Here's how the part is built. I have some questions about the finished solid (model axes, mm). A direction names the side the tool comes from. Give positions to 0.01 mm unless a question says otherwise; leave off trailing zeros. Loops run counter-clockwise (first coordinate to the right, second up) from the corner with the lowest first, then second, coordinate; pieces in that order, holes last.
Q1. For faces 5 (the face through (12, 0, 0)), 6 (the face through (-13.99, 5.99, 2.15)), 7 (the face through (10.907, -10.98, 5.898)), which set-ups out of +Z, -Z, +X, -X, +Y, -Y let a thin tool reach every point of the face, with its end or its side?
Q2. Thinking about a two-plate mould opening in Y: for faces 1 (the face through (0, 0, 7.5)), 2 (the face through (7, -13, 4.25)), 3 (the face through (-1, 13, 4.25)), 4 (the face through (-2.343, 17.847, 3.698)), which applies, pulls with the +Y half, pulls with the -Y half, needs draft (parallel to the pull), parting line crosses it, or undercut?
Q3. Suppose I cut it at D-D (z = -0.5). List the corners of the cut face in (x, y) for me.
Q4. I'm going to push flat-ended pins straight in: P1, Ø2.5, axis at x = 14.5, y = 4.5, coming from the +Z side; P2, Ø3, axis at y = -6, z = 6, coming from the +X side; P3, Ø1, axis at x = -12.5, y = -1.5, coming from the -Z side. Where does each tip first touch, or does it pass through?
Q5. Suppose I cut it at C-C (y = 14.5). List the corners of the cut face in (x, z) for me, and give its area (3 significant figures).
Q6. Suppose I cut it at B-B (y = 0). List the corners of the cut face in (x, z) for me.
Q7. I need wall thicknesses on probe 1 along Y at (x, z) = (0, 1.8); probe 2 along Y at (x, z) = (0, -4); probe 3 along Z at (x, y) = (14.5, -0.5). Which ranges of each line are inside material? Lowest first, please.
Q8. Suppose I cut it at A-A (x = 0). List the corners of the cut face in (y, z) for me.
```python
from build123d import *

# Parameters (mm, degrees)
SKETCH1_R           = 18
BOSS_EXTRUDE1_DEPTH = 7.5
SKETCH2_R           = 11.5
SKETCH2_R_2         = 4.5
BOSS_EXTRUDE2_DEPTH = 7.25
SKETCH3_R           = 1.524
CUT_EXTRUDE1_DEPTH  = 16.75
SKETCH4_R           = 2.5
CUT_EXTRUDE2_DEPTH  = 3.25


with BuildPart() as part:
    # Sketch1 → Boss-Extrude1 (new body)
    with BuildSketch(Plane.XY):
        Circle(SKETCH1_R)
    extrude(amount=BOSS_EXTRUDE1_DEPTH)

    # Sketch2 → Boss-Extrude2 (add)
    with BuildSketch(Plane(origin=(0, 0, 0), x_dir=(-1, 0, 0), z_dir=(0, 0, -1))):
        Circle(SKETCH2_R)
        Circle(SKETCH2_R_2, mode=Mode.SUBTRACT)
    extrude(amount=BOSS_EXTRUDE2_DEPTH)

    # Sketch3 → Cut-Extrude1 (cut)
    with BuildSketch(Plane.XY.offset(7.5)):
        with Locations((0, 14.5)):
            Circle(SKETCH3_R)
        with Locations((13.790319486, 4.480746418)):
            Circle(SKETCH3_R)
        with Locations((8.522886158, -11.730746418)):
            Circle(SKETCH3_R)
        with Locations((-8.522886158, -11.730746418)):
            Circle(SKETCH3_R)
        with Locations((-13.790319486, 4.480746418)):
            Circle(SKETCH3_R)
    extrude(amount=-CUT_EXTRUDE1_DEPTH, mode=Mode.SUBTRACT)

    # Sketch4 → Cut-Extrude2 (cut)
    with BuildSketch(Plane.XY.offset(7.5)):
        with Locations((0, 14.5)):
            Circle(SKETCH4_R)
        with Locations((13.790319486, 4.480746418)):
            Circle(SKETCH4_R)
        with Locations((8.522886158, -11.730746418)):
            Circle(SKETCH4_R)
        with Locations((-8.522886158, -11.730746418)):
            Circle(SKETCH4_R)
        with Locations((-13.790319486, 4.480746418)):
            Circle(SKETCH4_R)
    extrude(amount=-CUT_EXTRUDE2_DEPTH, mode=Mode.SUBTRACT)


solid = part.part
```
Solutions:
1. face 5: -Z
1. face 6: +Z, -Z
1. face 7: +Z
2. face 1: needs draft
2. face 2: undercut
2. face 3: undercut
2. face 4: parting line crosses it
3. outline: circle Ø23 at (0, 0); hole circle Ø9 at (0, 0)
4. P1: stops at z = 4.25
4. P2: stops at x = 17.43
4. P3: stops at z = 0
5. outline: (-10.67, 0) - (-1.52, 0) - (-1.52, 4.25) - (-2.5, 4.25) - (-2.5, 7.5) - (-10.67, 7.5) - close; (1.52, 0) - (10.67, 0) - (10.67, 7.5) - (2.5, 7.5) - (2.5, 4.25) - (1.52, 4.25) - close
5. area: 131 mm2
6. outline: (-18, 0) - (-11.5, 0) - (-11.5, -7.25) - (-4.5, -7.25) - (-4.5, 0) - (4.5, 0) - (4.5, -7.25) - (11.5, -7.25) - (11.5, 0) - (18, 0) - (18, 7.5) - (-18, 7.5) - close
7. probe 1: y = -18 to 12.98, 16.02 to 18
7. probe 2: y = -11.5 to -4.5, 4.5 to 11.5
7. probe 3: z = 0 to 7.5
8. outline: (-18, 0) - (-11.5, 0) - (-11.5, -7.25) - (-4.5, -7.25) - (-4.5, 0) - (4.5, 0) - (4.5, -7.25) - (11.5, -7.25) - (11.5, 0) - (12.98, 0) - (12.98, 4.25) - (12, 4.25) - (12, 7.5) - (-18, 7.5) - close; (16.02, 0) - (18, 0) - (18, 7.5) - (17, 7.5) - (17, 4.25) - (16.02, 4.25) - close
